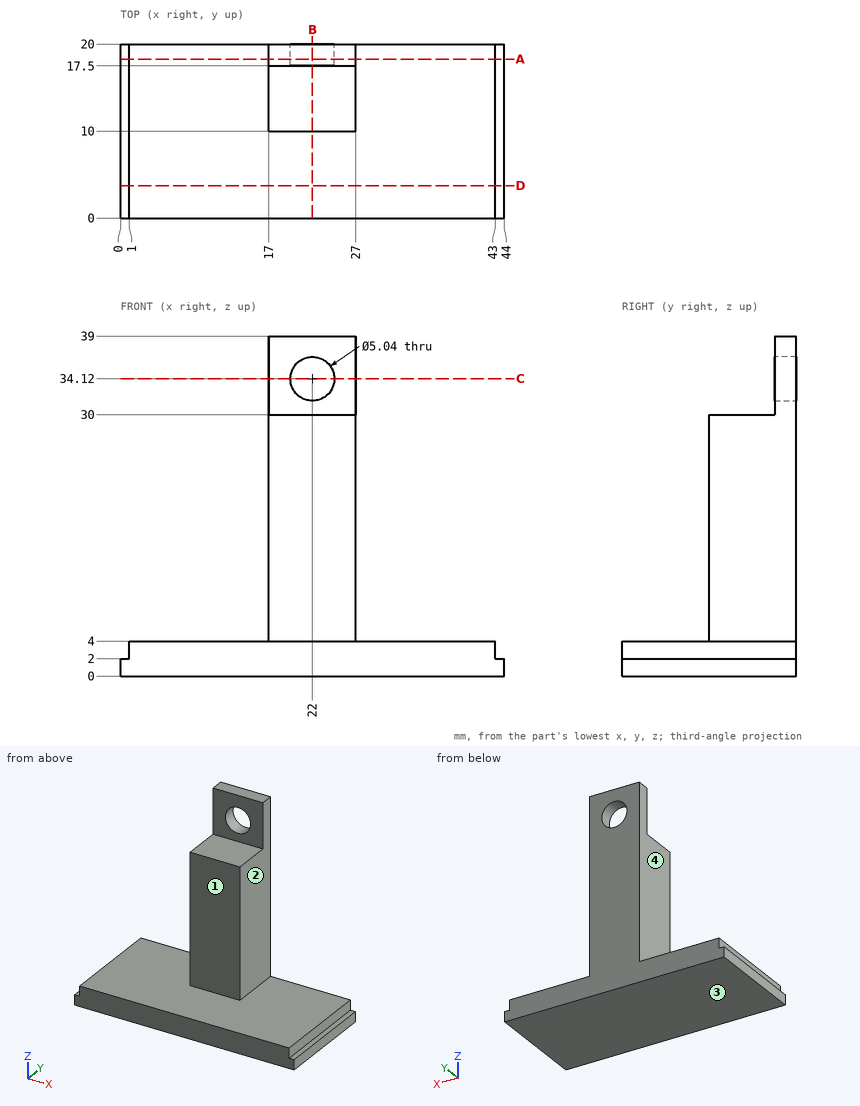
Geometry: see drawing. Coordinates: mm, zero at the bounding-box minimum. A direction names the side the tool comes from. Give positions to 0.01 mm unless a question says otherwise; leave off trailing zeros. Loops run counter-clockwise (first coordinate to the right, second up) from the corner with the lowest first, then second, coordinate; pieces in that order, holes last. Notation, with made-up numbers: (-22.5, 75.25) -> (31.5, 75.25) arc R21 ccw to (31.5, 102.25) -> close; hole circle Ø6 at (-13.75, 85). An arc over 180 degrees is marked (long way). Put each result on its own line as item: value.
1. Pin query (flat end, axial travel): P1, Ø2, axis at x = 17, z = 8.5, coming from the -Y side; P2, Ø1.1, axis at x = 0.5, y = 6, coming from the +Z side; P3, Ø0.8, axis at x = 43.5, y = 11.5, coming from the +Z side. Return the tip coordinate at first contact, or that it passes through.
Taken from the geometry:
P1: stops at y = 10
P2: stops at z = 4
P3: stops at z = 2
2. Cut plane D-D (y = 3.75). Return the cut outline in (x, z), plus the area to 3 significant figures.
Taken from the geometry:
outline: (0, 0) -> (44, 0) -> (44, 2) -> (43, 2) -> (43, 4) -> (1, 4) -> (1, 2) -> (0, 2) -> close
area: 172 mm2
3. Ray query, line 1 along X through (y, z) = (18.2, 34.12); line 2 along Y through (x, z) = (21.5, 8.5); line 3 along X through (y, z) = (12.5, 13.5). Return the intervals inside material, ascending. Write a range as [from, to].
Taken from the geometry:
line 1: x = [17, 19.48], [24.52, 27]
line 2: y = [10, 20]
line 3: x = [17, 27]
4. Cut plane A-A (y = 18.25). Return the cut outline in (x, z), plus the area to 3 significant figures.
Taken from the geometry:
outline: (0, 0) -> (44, 0) -> (44, 2) -> (43, 2) -> (43, 4) -> (27, 4) -> (27, 39) -> (17, 39) -> (17, 4) -> (1, 4) -> (1, 2) -> (0, 2) -> close; hole circle Ø5.04 at (22, 34.12)
area: 502 mm2
5. Set-up query: the marked faces 1, 2, 3 and 4. Return all of +Z, -Z, +X, -X, +Y, -Y with unobstructed straight access to the full face (end or side cutting, diameter ignored); none if empty.
Taken from the geometry:
face 1: +Z, +X, -X, -Y
face 2: +Z, +X, +Y, -Y
face 3: -Z, +X, -X, +Y, -Y
face 4: +Z, -X, +Y, -Y
6. Cut plane C-C (z = 34.12). Return the cut outline in (x, y), plus the area to 3 significant figures.
Taken from the geometry:
outline: (17, 17.5) -> (19.48, 17.5) -> (19.48, 20) -> (17, 20) -> close; (24.52, 17.5) -> (27, 17.5) -> (27, 20) -> (24.52, 20) -> close
area: 12.4 mm2
7. Cut plane B-B (x = 22). Return the cut outline in (y, z), plus the area to 3 significant figures.
Taken from the geometry:
outline: (0, 0) -> (20, 0) -> (20, 31.6) -> (17.5, 31.6) -> (17.5, 30) -> (10, 30) -> (10, 4) -> (0, 4) -> close; (17.5, 36.64) -> (20, 36.64) -> (20, 39) -> (17.5, 39) -> close
area: 350 mm2
